Could you check a few things on this drawing? It's one solid part, dimensions in mm from its lowest x, y, z. A direction names the side the tool comes from. Give positions to 0.01 mm unless a question says otherwise; leave off trailing zeros. Order: outer loops, then holes, each group sorted by start corner. A loop starts at its lowest first (then second) coordinate and runs counter-clockwise, first axis right, second up. Notation, with made-up numbers: M 3,-29 L 55,-29 A13 cw 55,-9 Z; hole C 40.5,29.5 d10. An arc over 180 degrees is marked long. Use one line per item in the form item = value. Start each with the question number.
1. Will these pins go through, and if not, where does the flat tip stop? P1, Ø2, axis at x = 14, y = 4.5, coming from the -Z side; P2, Ø1.5, axis at x = 14, z = 3, coming from the +Y side; P3, Ø3, axis at x = 9, z = 8.5, coming from the +Y side.
2. I want a section at B-B, the plane y = 0.5. List the corners of the cut face in (x, z) for me.
3. I need wall thicknesses on L1, parallel to Y at x = 1.95, z = 8.75; L2, parallel to Y at x = 14.5, z = 7.25; L3, parallel to X at y = 5, z = 6.25. Which ranges of each line are inside material? Lowest first, please.
4. I want a section at C-C, the plane y = 4.25. List the corners of the cut face in (x, z) for me, and give its area (3 significant figures).
5. I want a section at D-D, the plane z = 8.25. List the corners of the cut face in (x, y) for me.
6. We'd pull the mould along Y, two halves only. Please class the marked faces 4, 5 and 6: +Y half, -Y half, draft (parallel to the pull), parting line (faces both ways), or undercut.
7. For the marked faces 1, 2 and 3, which set-ups out of +Z, -Z, +X, -X, +Y, -Y let a thin tool reach every point of the face, with its end or its side?
8. I want a section at A-A, the plane x = 2. List the corners of the cut face in (y, z) for me, and give its area (3 significant figures).
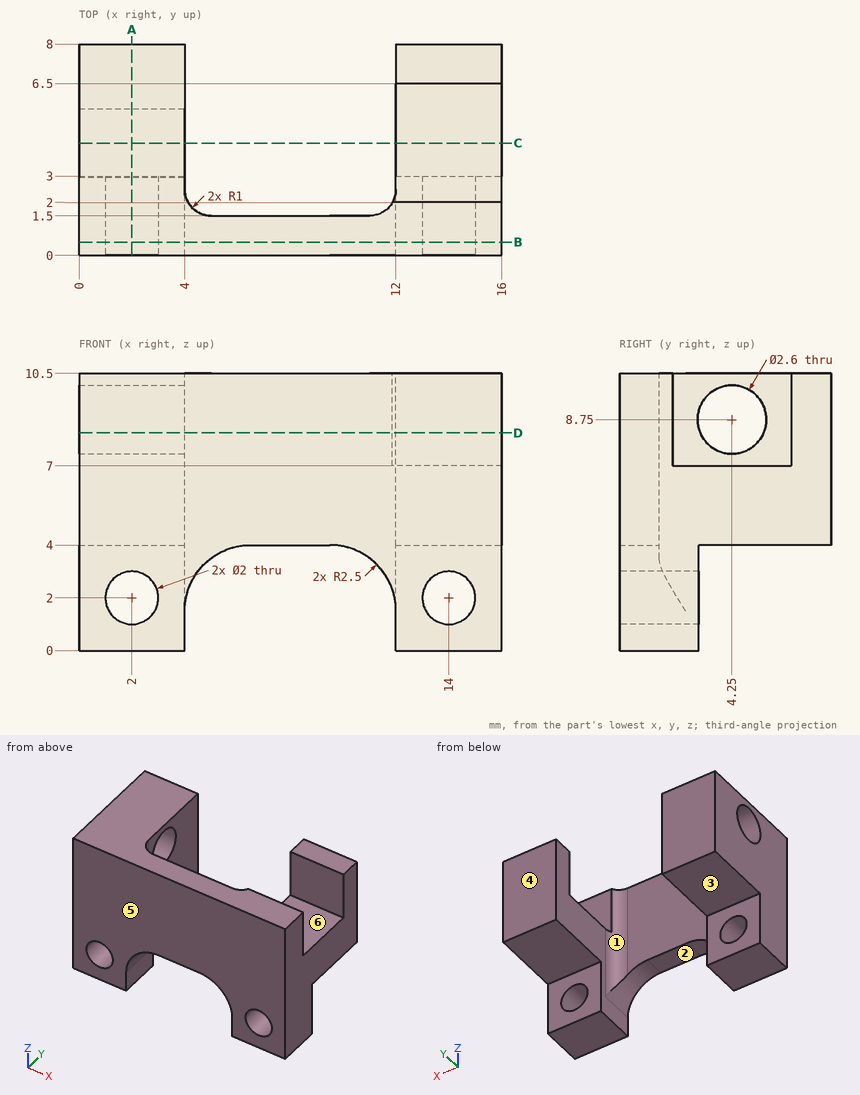
Check result:
q1.P1 = 4
q1.P2 = 3
q1.P3 = 1.5
q2.outline = M 0,0 L 4,0 L 4,1.5 A2.5 cw 6.5,4 L 9.5,4 A2.5 cw 12,1.5 L 12,0 L 16,0 L 16,10.5 L 0,10.5 Z; hole C 2,2 d2; hole C 14,2 d2
q3.L1 = 0 to 2.95, 5.55 to 8
q3.L2 = 0 to 2, 6.5 to 8
q3.L3 = 0 to 4, 12 to 16
q4.outline = M 0,4 L 4,4 L 4,7.45 L 0,7.45 Z; M 0,10.05 L 4,10.05 L 4,10.5 L 0,10.5 Z; M 12,4 L 16,4 L 16,7 L 12,7 Z
q4.area = 27.6 mm2
q5.outline = M 0,0 L 16,0 L 16,2 L 11.87,2 A1 cw 11,1.5 L 5,1.5 A1 cw 4,2.5 L 4,3.05 L 0,3.05 Z; M 0,5.45 L 4,5.45 L 4,8 L 0,8 Z; M 12,6.5 L 16,6.5 L 16,8 L 12,8 Z
q6.face_4 = +Y half
q6.face_5 = -Y half
q6.face_6 = undercut
q7.face_1 = +Z, -Z, +Y
q7.face_2 = -Z, +Y, -Y
q7.face_3 = -Z, +X, -X, +Y
q8.outline = M 0,0 L 3,0 L 3,1 L 0,1 Z; M 0,3 L 3,3 L 3,4 L 8,4 L 8,10.5 L 0,10.5 Z; hole C 4.25,8.75 d2.6
q8.area = 52.7 mm2
